```python
from build123d import *

# Parameters (mm, degrees)
SKETCH1_R           = 6.9
BOSS_EXTRUDE1_DEPTH = 6.8
SKETCH2_R           = 1
CUT_EXTRUDE1_DEPTH  = 2
SKETCH3_R           = 0.35
BOSS_EXTRUDE2_DEPTH = 4.5


with BuildPart() as part:
    # Sketch1 → Boss-Extrude1 (new body)
    with BuildSketch(Plane.XY):
        Circle(SKETCH1_R)
    extrude(amount=BOSS_EXTRUDE1_DEPTH)

    # Sketch2 → Cut-Extrude1 (cut)
    with BuildSketch(Plane.XY.offset(6.8)):
        Circle(SKETCH2_R)
    extrude(amount=-CUT_EXTRUDE1_DEPTH, mode=Mode.SUBTRACT)

    # Sketch3 → Boss-Extrude2 (add)
    with BuildSketch(Plane(origin=(0, 0, 0), x_dir=(-1, 0, 0), z_dir=(0, 0, -1))):
        with Locations(Location((0, 3.8, 0), (0, 0, 180))):
            Circle(SKETCH3_R)
        with Locations(Location((0, -3.8, 0), (0, 0, 180))):
            Circle(SKETCH3_R)
    extrude(amount=BOSS_EXTRUDE2_DEPTH)


solid = part.part
```
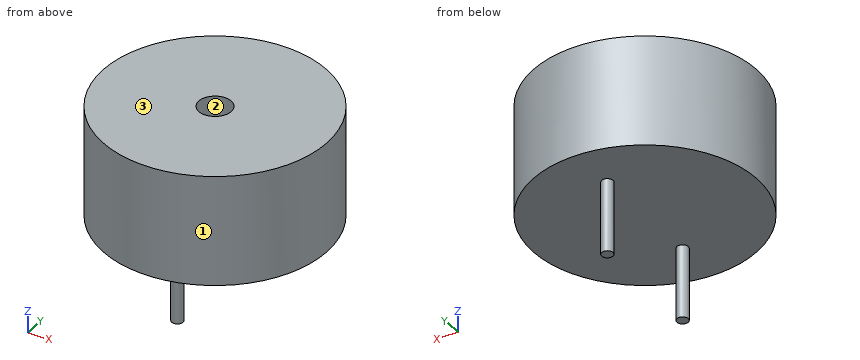
Geometry check sheet. Reference: the model listing, model coordinates, mm. Face numbers are marked on the shaded views. Coordinates: 2 decimals unless noted, no trailing zeros. Order: outer loops, then holes, each group sorted by start corner. A loop starts at its lowest first (then second) coordinate and runs counter-clockwise, first axis right, second up.
Item 1: Section check B-B (z = -0.75). Enter the section's corners in (x, y), plus the area to 3 significant figures.
Item 2: Section check A-A (y = 0). Enter the section's corners in (x, z).
Item 3: Section check D-D (z = 5.75). Enter the section's corners in (x, y).
Item 4: Mould release check, pull along Y, two halves, no side actions. Record for the marked faces 1, 2 and 3: released by +Y, released by -Y, zero draft, split by the parting line, or undercut.
Item 5: Section check C-C (x = 0). Enter the section's corners in (y, z), plus the area to 3 significant figures.
Item 6: Scan lines: line 1 along Y through (x, z) = (0, 5.9); line 2 along Z through (x, y) = (1, -1.25); line 3 along X through (y, z) = (3, 0.25). Record each from-to range of solid material in increasing order.
Item 7: Depth check by flat-ended pin: pin 1 (1 mm diameter, centred on x = -1, z = -2.5, fed in from -Y); pin 2 (1 mm diameter, centred on y = -2.5, z = 2, fed in from -X); pin 3 (1 mm diameter, centred on x = -3.5, y = 1.5, fed in from -Z); pin 4 (4 mm diameter, centred on x = 3.5, z = 0.5, fed in from -Y) (3 decimals). Enter the tip coordinate at first touch or a pass-through.
Check sheet entries:
1. outline: circle Ø0.7 at (0, -3.8); circle Ø0.7 at (0, 3.8)
1. area: 0.770 mm2
2. outline: (-6.9, 0) - (6.9, 0) - (6.9, 6.8) - (1, 6.8) - (1, 4.8) - (-1, 4.8) - (-1, 6.8) - (-6.9, 6.8) - close
3. outline: circle Ø13.8 at (0, 0); hole circle Ø2 at (0, 0)
4. face 1: split by the parting line
4. face 2: undercut
4. face 3: zero draft
5. outline: (-6.9, 0) - (-4.15, 0) - (-4.15, -4.5) - (-3.45, -4.5) - (-3.45, 0) - (3.45, 0) - (3.45, -4.5) - (4.15, -4.5) - (4.15, 0) - (6.9, 0) - (6.9, 6.8) - (1, 6.8) - (1, 4.8) - (-1, 4.8) - (-1, 6.8) - (-6.9, 6.8) - close
5. area: 96.1 mm2
6. line 1: y = -6.9 to -1, 1 to 6.9
6. line 2: z = 0 to 6.8
6. line 3: x = -6.21 to 6.21
7. pin 1: passes through
7. pin 2: stops at x = -6.6
7. pin 3: stops at z = 0
7. pin 4: stops at y = -6.735
